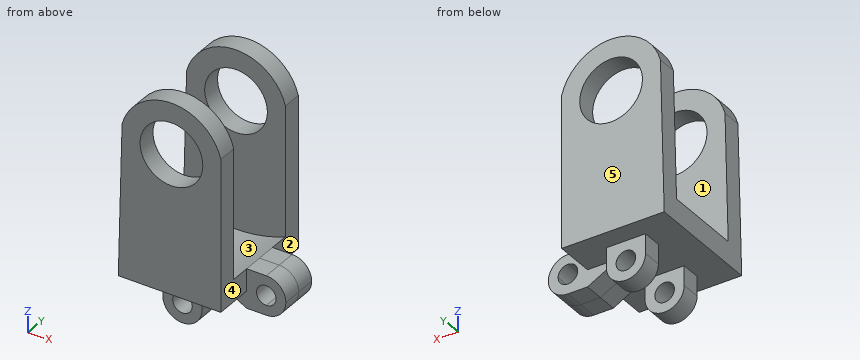
from build123d import *

# Parameters (mm, degrees)
SKETCH1_R           = 16.51
SKETCH1_R_2         = 10.16
BOSS_EXTRUDE1_DEPTH = 38.1
CUT_EXTRUDE1_START  = 6.35
SKETCH1_3_R         = 16.51
SKETCH1_3_R_2       = 10.16
CUT_EXTRUDE1_DEPTH  = 25.4
CUT_EXTRUDE2_REACH  = 66.365
BOSS_EXTRUDE2_START = 6.35
SKETCH7_R           = 3.175
BOSS_EXTRUDE2_DEPTH = 6.35
BOSS_EXTRUDE3_DEPTH = 6.35


with BuildPart() as part:
    # Sketch1 → Boss-Extrude1 (new body)
    # profile 1 of 4: a face of its own
    with BuildSketch(Plane(origin=(0, 0, 0), x_dir=(1, 0, 0), z_dir=(0, 1, 0))):
        with BuildLine():
            Line((-25.4, 45.234068682), (-25.4, 32.534068682))
            ThreePointArc((-25.4, 32.534068682), (0, 41.275), (25.4, 32.534068682))
            Line((25.4, 32.534068682), (25.4, 45.234068682))
            Line((25.4, 45.234068682), (-25.4, 45.234068682))
        make_face()
    # profile 2 of 4: a face of its own
    with BuildSketch(Plane(origin=(0, 0, 0), x_dir=(1, 0, 0), z_dir=(0, 1, 0))):
        with BuildLine():
            ThreePointArc((25.4, 32.534068682), (0, 41.275), (-25.4, 32.534068682))
            Line((-25.4, 32.534068682), (25.4, 32.534068682))
        make_face()
    # profile 3 of 4: a face of its own
    with BuildSketch(Plane(origin=(0, 0, 0), x_dir=(1, 0, 0), z_dir=(0, 1, 0))):
        with BuildLine():
            Line((25.4, 32.534068682), (-25.4, 32.534068682))
            Line((-25.4, 32.534068682), (-15.991186592, -4.106342823))
            ThreePointArc((-15.991186592, -4.106342823), (-2.069493823, 16.379783128), (16.51, 0))
            ThreePointArc((16.51, 0), (16.379783128, -2.069493823), (15.991186592, -4.106342823))
            Line((15.991186592, -4.106342823), (25.4, 32.534068682))
        make_face()
    # profile 4 of 4: a face of its own
    with BuildSketch(Plane(origin=(0, 0, 0), x_dir=(1, 0, 0), z_dir=(0, 1, 0))):
        Circle(SKETCH1_R)
        with Locations(Location((0, 0, 0), (0, 0, 90))):
            Circle(SKETCH1_R_2, mode=Mode.SUBTRACT)
    extrude(amount=BOSS_EXTRUDE1_DEPTH)

    # Sketch1<3> → Cut-Extrude1 (cut)
    # profile 1 of 3: a face of its own
    with BuildSketch(Plane(origin=(0, 0, 0), x_dir=(1, 0, 0), z_dir=(0, 1, 0)).offset(CUT_EXTRUDE1_START)):
        with BuildLine():
            Line((25.4, 32.534068682), (-25.4, 32.534068682))
            Line((-25.4, 32.534068682), (-15.991186592, -4.106342823))
            ThreePointArc((-15.991186592, -4.106342823), (-2.069493823, 16.379783128), (16.51, 0))
            ThreePointArc((16.51, 0), (16.379783128, -2.069493823), (15.991186592, -4.106342823))
            Line((15.991186592, -4.106342823), (25.4, 32.534068682))
        make_face()
    # profile 2 of 3: a face of its own
    with BuildSketch(Plane(origin=(0, 0, 0), x_dir=(1, 0, 0), z_dir=(0, 1, 0)).offset(CUT_EXTRUDE1_START)):
        with BuildLine():
            ThreePointArc((25.4, 32.534068682), (0, 41.275), (-25.4, 32.534068682))
            Line((-25.4, 32.534068682), (25.4, 32.534068682))
        make_face()
    # profile 3 of 3: a face of its own
    with BuildSketch(Plane(origin=(0, 0, 0), x_dir=(1, 0, 0), z_dir=(0, 1, 0)).offset(CUT_EXTRUDE1_START)):
        Circle(SKETCH1_3_R)
        with Locations(Location((0, 0, 0), (0, 0, 90))):
            Circle(SKETCH1_3_R_2, mode=Mode.SUBTRACT)
    extrude(amount=CUT_EXTRUDE1_DEPTH, mode=Mode.SUBTRACT)

    # Cut-Extrude2: up to this face of the body (flat: up to its plane)
    cut_extrude2_end = Plane(part.part.faces().sort_by_distance((0, 0, -21.591993841))[0])
    # Sketch5 → Cut-Extrude2 (cut, up to the picked face)
    with BuildSketch(Plane(origin=(0, 38.1, 0), x_dir=(1, 0, 0), z_dir=(0, 1, 0)), mode=Mode.PRIVATE) as cut_extrude2_sk1:
        Polygon((15.991186592, 45.234068682), (15.991186592, -4.106342823), (25.4, 32.534068682), (25.4, 45.234068682), align=None)
    cut_extrude2_tool1 = split(extrude(cut_extrude2_sk1.sketch, amount=-CUT_EXTRUDE2_REACH, mode=Mode.PRIVATE), bisect_by=cut_extrude2_end, keep=Keep.BOTH, mode=Mode.PRIVATE)
    # Sketch5 → Cut-Extrude2 (cut, up to the picked face)
    with BuildSketch(Plane(origin=(0, 38.1, 0), x_dir=(1, 0, 0), z_dir=(0, 1, 0)), mode=Mode.PRIVATE) as cut_extrude2_sk2:
        Polygon((-25.4, 32.534068682), (-15.991186592, -4.106342823), (-17.209379635, 45.234068682), (-25.4, 45.234068682), align=None)
    cut_extrude2_tool2 = split(extrude(cut_extrude2_sk2.sketch, amount=-CUT_EXTRUDE2_REACH, mode=Mode.PRIVATE), bisect_by=cut_extrude2_end, keep=Keep.BOTH, mode=Mode.PRIVATE)
    add(cut_extrude2_tool1.solids().sort_by(Axis((19.769469, 38.1, -27.920679), (0, -1, 0)))[0], mode=Mode.SUBTRACT)
    add(cut_extrude2_tool2.solids().sort_by(Axis((-20.156564, 38.1, -27.821204), (0, -1, 0)))[0], mode=Mode.SUBTRACT)

    # Sketch7 → Boss-Extrude2 (add)
    with BuildSketch(Plane(origin=(0, 19.05, 0), x_dir=(1, 0, 0), z_dir=(0, 1, 0)).offset(BOSS_EXTRUDE2_START)):
        with BuildLine():
            Line((5.740903479, 45.234068682), (5.740903479, 51.584068682))
            ThreePointArc((5.740903479, 51.584068682), (-0.609096521, 57.934068682), (-6.959096521, 51.584068682))
            Line((-6.959096521, 51.584068682), (-6.959096521, 45.234068682))
            Line((-6.959096521, 45.234068682), (-0.609096521, 45.234068682))
            Line((-0.609096521, 45.234068682), (5.740903479, 45.234068682))
        make_face()
        with Locations(Location((-0.609096521, 51.584068682, 0), (0, 0, 270))):
            Circle(SKETCH7_R, mode=Mode.SUBTRACT)
    boss_extrude2 = extrude(amount=BOSS_EXTRUDE2_DEPTH)

    # Sketch8 → Boss-Extrude3 (add)
    with BuildSketch(Plane(origin=(0, 19.05, 0), x_dir=(1, 0, 0), z_dir=(0, 1, 0))):
        with BuildLine():
            ThreePointArc((15.991186592, 44.401380742), (17.851058531, 39.911252682), (22.341186592, 38.051380742))
            Line((22.341186592, 38.051380742), (22.341186592, 41.226380742))
            ThreePointArc((22.341186592, 41.226380742), (19.166186592, 44.401380742), (22.341186592, 47.576380742))
            Line((22.341186592, 47.576380742), (22.341186592, 50.751380742))
            ThreePointArc((22.341186592, 50.751380742), (17.851058531, 48.891508803), (15.991186592, 44.401380742))
        make_face()
        with BuildLine():
            Line((22.341186592, 41.226380742), (22.341186592, 38.051380742))
            ThreePointArc((22.341186592, 38.051380742), (26.831314653, 39.911252682), (28.691186592, 44.401380742))
            ThreePointArc((28.691186592, 44.401380742), (26.831314653, 48.891508803), (22.341186592, 50.751380742))
            Line((22.341186592, 50.751380742), (22.341186592, 47.576380742))
            ThreePointArc((22.341186592, 47.576380742), (24.586250622, 46.646444772), (25.516186592, 44.401380742))
            ThreePointArc((25.516186592, 44.401380742), (24.586250622, 42.156316712), (22.341186592, 41.226380742))
        make_face()
        with BuildLine():
            ThreePointArc((15.991186592, 44.401380742), (17.851058531, 39.911252682), (22.341186592, 38.051380742))
            Line((22.341186592, 38.051380742), (22.341186592, 41.226380742))
            ThreePointArc((22.341186592, 41.226380742), (19.166186592, 44.401380742), (22.341186592, 47.576380742))
            Line((22.341186592, 47.576380742), (22.341186592, 50.751380742))
            ThreePointArc((22.341186592, 50.751380742), (17.851058531, 48.891508803), (15.991186592, 44.401380742))
        make_face()
        with BuildLine():
            Line((22.341186592, 41.226380742), (22.341186592, 38.051380742))
            ThreePointArc((22.341186592, 38.051380742), (26.831314653, 39.911252682), (28.691186592, 44.401380742))
            ThreePointArc((28.691186592, 44.401380742), (26.831314653, 48.891508803), (22.341186592, 50.751380742))
            Line((22.341186592, 50.751380742), (22.341186592, 47.576380742))
            ThreePointArc((22.341186592, 47.576380742), (24.586250622, 46.646444772), (25.516186592, 44.401380742))
            ThreePointArc((25.516186592, 44.401380742), (24.586250622, 42.156316712), (22.341186592, 41.226380742))
        make_face()
        with BuildLine():
            Line((15.991186592, 45.234068682), (15.991186592, 44.401380742))
            ThreePointArc((15.991186592, 44.401380742), (17.851058531, 48.891508803), (22.341186592, 50.751380742))
            Line((22.341186592, 50.751380742), (15.991186592, 50.751380742))
            Line((15.991186592, 50.751380742), (15.991186592, 45.234068682))
        make_face()
        with BuildLine():
            Line((15.991186592, 44.401380742), (15.991186592, 38.051380742))
            Line((15.991186592, 38.051380742), (22.341186592, 38.051380742))
            ThreePointArc((22.341186592, 38.051380742), (17.851058531, 39.911252682), (15.991186592, 44.401380742))
        make_face()
        Polygon((15.991186592, 50.751380742), (15.991186592, 45.234068682), (5.740903479, 45.234068682), align=None)
    boss_extrude3 = extrude(amount=BOSS_EXTRUDE3_DEPTH)

    # Mirror1: Boss-Extrude2, Boss-Extrude3 across plane
    add(boss_extrude2.mirror(Plane.ZX.offset(19.05)))
    add(boss_extrude3.mirror(Plane.ZX.offset(19.05)))


solid = part.part
Part model, mm, in its own coordinate system. Face numbers are marked on the shaded views. A direction names the side the tool comes from. Give positions to 0.01 mm unless a question says otherwise; leave off trailing zeros. Loops run counter-clockwise (first coordinate to the right, second up) from the corner with the lowest first, then second, coordinate; pieces in that order, holes last. Notation, with made-up numbers: M 20.25,22 L 49.25,22 A31 ccw 49.25,49 Z; hole C 88.25,62 d2. An arc over 180 degrees is marked long. Put each result on its own line as item: value. Start each with the question number.
1) Pull direction X, two halves, no side cores. Call the marked faces 3, 4 and 5: +X half, -X half, draft (parallel to the pull), parting line (faces both ways), or undercut.
2) Probe probe 1 along Y at (x, z) = (-5, -24.5); probe 2 along X at (y, z) = (36, 0); probe 3 along X at (y, z) = (23.5, -46). List the from-to ranges inside material, lowest first.
3) Saw through at B-B (z = -23.5). List the corners of the cut face in (x, y), then the cut area to 3 significant figures.
4) Saw through at D-D (z = 9). List the corners of the cut face in (x, y), then the cut area to 3 significant figures.
5) Saw through at A-A (y = 15.5). List the corners of the cut face in (x, z) (3 decimals).
6) Saw through at C-C (x = 8.5). List the corners of the cut face in (y, z), then the cut area to 3 significant figures.
7) Flat gauge pins, fed straight in: pin 1 (10 mm diameter, centred on x = -0.5, z = -52.5, fed in from -Y); pin 2 (6 mm diameter, centred on x = -6.5, y = 13, fed in from -Z); pin 3 (4 mm diameter, centred on x = 0.5, z = -49, fed in from +Y). Where does each tip first touch, or does it go through?
8) 3-axis set-ups, long thin cutter, end or side, ignore diameter. For the marked faces 1 and 2: which of +Z, -Z, +X, -X, +Y, -Y reach the whole face in a straight line?
Numbers:
1. face 3: undercut
1. face 4: +X half
1. face 5: draft
2. probe 1: 0 to 6.35, 31.75 to 38.1
2. probe 2: -16.09 to -10.16, 10.16 to 15.99
2. probe 3: 7.16 to 19.6, 25.08 to 28.49
3. outline: M -16.67,0 L 15.99,0 L 15.99,6.35 L -16.67,6.35 Z; M -16.67,31.75 L 15.99,31.75 L 15.99,38.1 L -16.67,38.1 Z
3. area: 415 mm^2
4. outline: M -13.84,0 L -4.71,0 L -4.71,6.35 L -13.84,6.35 Z; M -13.84,31.75 L -4.71,31.75 L -4.71,38.1 L -13.84,38.1 Z; M 4.71,0 L 13.84,0 L 13.84,6.35 L 4.71,6.35 Z; M 4.71,31.75 L 13.84,31.75 L 13.84,38.1 L 4.71,38.1 Z
4. area: 232 mm^2
5. outline: M -17.209,-45.234 L 5.741,-45.234 L 15.991,-50.751 L 22.341,-50.751 A6.35 ccw 22.341,-38.051 L 15.991,-38.051 A41.275 cw -17.021,-37.602 Z; hole C 22.341,-44.401 d6.35
6. outline: M 0,-45.23 L 12.7,-45.23 L 12.7,-46.72 L 25.4,-46.72 L 25.4,-45.23 L 38.1,-45.23 L 38.1,-5.57 L 31.75,-5.57 L 31.75,-40.39 L 6.35,-40.39 L 6.35,-5.57 L 0,-5.57 Z; M 0,5.57 L 6.35,5.57 L 6.35,14.15 L 0,14.15 Z; M 31.75,5.57 L 38.1,5.57 L 38.1,14.15 L 31.75,14.15 Z
6. area: 755 mm^2
7. pin 1: y = 6.35
7. pin 2: z = -57.23
7. pin 3: y = 31.75
8. face 1: +Z
8. face 2: +Z, -Z, +X, +Y
